from build123d import *

# Parameters (mm, degrees)
SKETCH1_R           = 2
BOSS_EXTRUDE1_DEPTH = 5
SKETCH2_R           = 3
BOSS_EXTRUDE2_DEPTH = 26
SKETCH3_R           = 2
BOSS_EXTRUDE3_DEPTH = 5
SKETCH4_R           = 0.75
CUT_EXTRUDE1_DEPTH  = 2.5


with BuildPart() as part:
    # Sketch1 → Boss-Extrude1 (new body)
    with BuildSketch(Plane(origin=(0, 0, 0), x_dir=(0, 0, -1), z_dir=(1, 0, 0))):
        Circle(SKETCH1_R)
    extrude(amount=BOSS_EXTRUDE1_DEPTH)

    # Sketch2 → Boss-Extrude2 (add)
    with BuildSketch(Plane(origin=(5, 0, 0), x_dir=(0, 0, -1), z_dir=(1, 0, 0))):
        with Locations(Location((0, 0, 0), (0, 0, 180))):
            Circle(SKETCH2_R)
    extrude(amount=BOSS_EXTRUDE2_DEPTH)

    # Sketch3 → Boss-Extrude3 (add)
    with BuildSketch(Plane(origin=(31, 0, 0), x_dir=(0, 0, -1), z_dir=(1, 0, 0))):
        Circle(SKETCH3_R)
    extrude(amount=BOSS_EXTRUDE3_DEPTH)

    # Sketch4 → Cut-Extrude1 (cut, symmetric)
    with BuildSketch(Plane.XY):
        with Locations((33.5, 0)):
            Circle(SKETCH4_R)
        with Locations((2.5, 0)):
            Circle(SKETCH4_R)
    extrude(amount=CUT_EXTRUDE1_DEPTH, both=True, mode=Mode.SUBTRACT)


solid = part.part
Model file for the job. Use its own axes, mm. A direction names the side the tool comes from. Round coordinates to 2 decimals unless told otherwise and drop trailing zeros. Order: outer loops, then holes, each group sorted by start corner. A loop starts at its lowest first (then second) coordinate and runs counter-clockwise, first axis right, second up.
(1) Pull direction Y, two halves, no side cores. Call faces 1 (the face through (31, 1, 2)), 2 (the face through (34.215, 0.225, 0.028)), 3 (the face through (33.465, -1.774, -0.923)): released by +Y, released by -Y, zero draft, split by the parting line, or undercut.
(2) Band-saw the part on D-D (y = 1.7). List the corners of the cut face in (x, z), then the cut area to 3 significant figures.
(3) 3-axis set-ups, long thin cutter, end or side, ignore diameter. For faces 4 (the face through (5, 1, 2)), 5 (the face through (0, 0, 0)): which of +Z, -Z, +X, -X, +Y, -Y reach the whole face in a straight line?
(4) Band-saw the part on B-B (z = 0). List the corners of the cut face in (x, y).
(5) Drill centre lines: line 1 (X direction, y = 0, z = 0.35); line 2 (Y direction, x = 2.5, z = 1.15); line 3 (X direction, y = -1.55, z = -2.25). Where is each one in solid material? Low to high.
(6) Band-saw the part on C-C (x = 33.5). List the corners of the cut face in (y, z).
(7) Band-saw the part on A-A (y = 0). List the corners of the cut face in (x, z).
(8) Pin check, flat tips, straight feed: pin 1 (1.2 mm diameter, centred on x = 33.5, y = 0, fed in from +Z); pin 2 (3 mm diameter, centred on x = 10, z = -1, fed in from -Y); pin 3 (1 mm diameter, centred on y = -1, z = 2.5, fed in from +X); pin 4 (2 mm diameter, centred on x = 2.5, y = 0, fed in from -Z). Stop position of each tip, or through.
Verdict:
1. face 1: zero draft
1. face 2: undercut
1. face 3: split by the parting line
2. outline: (0, -1.05) - (5, -1.05) - (5, -2.47) - (31, -2.47) - (31, -1.05) - (36, -1.05) - (36, 1.05) - (31, 1.05) - (31, 2.47) - (5, 2.47) - (5, 1.05) - (0, 1.05) - close
2. area: 150 mm2
3. face 4: -X
3. face 5: +Z, -Z, -X, +Y, -Y
4. outline: (0, -2) - (5, -2) - (5, -3) - (31, -3) - (31, -2) - (36, -2) - (36, 2) - (31, 2) - (31, 3) - (5, 3) - (5, 2) - (0, 2) - close; hole circle Ø1.5 at (2.5, 0); hole circle Ø1.5 at (33.5, 0)
5. line 1: x = 0 to 1.75, 3.25 to 32.75, 34.25 to 36
5. line 2: y = -1.64 to -0.75, 0.75 to 1.64
5. line 3: x = 5 to 31
6. outline: (-0.75, -1.85) - (-0.75, 1.85) arc R2 ccw to start; (0.75, -1.85) arc R2 ccw to (0.75, 1.85) - close
7. outline: (0, -2) - (1.75, -2) - (1.75, 2) - (0, 2) - close; (3.25, -2) - (5, -2) - (5, -3) - (31, -3) - (31, -2) - (32.75, -2) - (32.75, 2) - (31, 2) - (31, 3) - (5, 3) - (5, 2) - (3.25, 2) - close; (34.25, -2) - (36, -2) - (36, 2) - (34.25, 2) - close
8. pin 1: passes through
8. pin 2: stops at y = -3
8. pin 3: stops at x = 31
8. pin 4: stops at z = -2
